from build123d import *

# Parameters (mm, degrees)
EXTRUDE_1_DEPTH     = 45
SKETCH_3_R          = 2
CUT_EXTRUDE_2_DEPTH = 90
SKETCH_4_R          = 2
CUT_EXTRUDE_3_DEPTH = 90
SKETCH_5_R          = 20
CUT_EXTRUDE_4_DEPTH = 90


with BuildPart() as part:
    # 草图1 → 凸台-拉伸1 (new, symmetric)
    with BuildSketch(Plane(origin=(0, 0, 0), x_dir=(1, 0, 0), z_dir=(0, 1, 0))):
        Polygon((0, 0), (0, 120), (160, 280), (157.171572875, 282.828427125), (-4, 121.656854249), (-4, 0), align=None)
    extrude(amount=EXTRUDE_1_DEPTH, both=True)

    # 草图3 → 切除-拉伸2 (cut)
    with BuildSketch(Plane.ZY.offset(4)):
        with Locations((-70, -36)):
            Circle(SKETCH_3_R)
    cut_extrude_2 = extrude(amount=-CUT_EXTRUDE_2_DEPTH, mode=Mode.SUBTRACT)

    # 草图4 → 切除-拉伸3 (cut)
    with BuildSketch(Plane(origin=(-60, 0, -60), x_dir=(0.7071067811865487, 0, -0.7071067811865465), z_dir=(0.7071067811865465, 0, 0.7071067811865487))):
        with Locations((124.852813742, -36)):
            Circle(SKETCH_4_R)
        with Locations((251.126983722, -36)):
            Circle(SKETCH_4_R)
    cut_extrude_3 = extrude(amount=-CUT_EXTRUDE_3_DEPTH, mode=Mode.SUBTRACT)

    # 镜向1: 切除-拉伸2, 切除-拉伸3 across plane
    add(cut_extrude_2.mirror(Plane.ZX), mode=Mode.SUBTRACT)
    add(cut_extrude_3.mirror(Plane.ZX), mode=Mode.SUBTRACT)

    # 草图5 → 切除-拉伸4 (cut)
    with BuildSketch(Plane.ZY.offset(4)):
        with Locations((-55, 0)):
            Circle(SKETCH_5_R)
    extrude(amount=-CUT_EXTRUDE_4_DEPTH, mode=Mode.SUBTRACT)


solid = part.part
The listing builds one solid part. Answer for the finished solid, in the listing's coordinates (mm). A direction names the side the tool comes from. Round coordinates to 2 decimals unless told otherwise and drop trailing zeros. Loops run counter-clockwise (first coordinate to the right, second up) from the corner with the lowest first, then second, coordinate; pieces in that order, holes last. Notation, with made-up numbers: M 78.5,77 L 109.5,77 A29 cw 109.5,111 Z; hole C 59.25,-6 d10. An arc over 180 degrees is marked long. Write each question's results on one line, items separated by ' | '. Start each with the question number.
1) Each of these flat-tipped pins is pushed along its axis until it touches: pin 1 (2 mm diameter, centred on x = 82.5, y = 30.5, fed in from +Z); pin 2 (2.5 mm diameter, centred on y = 36, z = -70, fed in from +X); pin 3 (6 mm diameter, centred on x = 83, y = 30.5, fed in from -Z); pin 4 (1.5 mm diameter, centred on y = 17, z = -78, fed in from +X). Where does it stop, or does it pass through?
2) Find section C-C on x = 131. Write down the section's boundary in (y, z).
3) Straight lines are drawn through the part: probe 1 along Y at (x, z) = (-1.55, -55); probe 2 along Y at (x, z) = (-3, -70); probe 3 along X at (y, z) = (-20.5, -39). For each, find the intervals that lie inside material, in ascending order.
4) Find section A-A on z = -55. Write down the section's boundary in (x, y).
5) Find section B-B on z = -116.5. Write down the section's boundary in (x, y), plus the area to 3 significant figures.
6) Determine the mould class of faces 1 (the cylindrical face through (27.5, -37.8, -150.3)), 2 (the flat face through (29, -45, -153)), 3 (the flat face through (29, 45, -153)), 4 (the flat face through (79, 1, -199)) for opening direction Y: pulls with the +Y half, pulls with the -Y half, needs draft (parallel to the pull), parting line crosses it, or undercut.
7) Which of the six approach directions +Z, -Z, +X, -X, +Y, -Y give full straight-line access (tool end or side, diameter ignored) to faces 5 (the flat face through (0, 11, -72)), 6 (the cylindrical face through (115.87, -37.95, -238.66))?
Final values:
1) pin 1: z = -201.5 | pin 2: through | pin 3: z = -211.66 | pin 4: x = 0
2) outline: M -45,-256.66 L 45,-256.66 L 45,-251 L -45,-251 Z
3) probe 1: -45 to -20, 20 to 45 | probe 2: -45 to -38, -34 to -13.23, 13.23 to 34, 38 to 45 | probe 3: -4 to 0
4) outline: M -4,-45 L 0,-45 L 0,-20 L -4,-20 Z; M -4,20 L 0,20 L 0,45 L -4,45 Z
5) outline: M -4,-45 L 0,-45 L 0,45 L -4,45 Z | area: 360 mm²
6) face 1: undercut | face 2: pulls with the -Y half | face 3: pulls with the +Y half | face 4: needs draft
7) face 5: +Z, +X, +Y, -Y | face 6: none
